from build123d import *

# Parameters (mm, degrees)
F1_DEPTH  = 49
F2_W      = 51.5
F2_H      = 79
F3_DEPTH  = 2
F2_R      = 1.5
F2_R_2    = 4.5
F4_DEPTH  = 7.3
F6_DEPTH  = 2
F8_DEPTH  = 2
F2_R_3    = 5
F9_DEPTH  = 2
F11_DEPTH = 2
F12_W     = 8.5
F12_H     = 55
F13_DEPTH = 40
F14_R     = 1.99999
F15_W     = 2
F15_H     = 19.5
F16_DEPTH = 20
F17_W     = 2
F17_H     = 19.5
F18_DEPTH = 20
F19_R     = 5
F20_DEPTH = 2
F21_R     = 2.5
F22_DEPTH = 7.5
F21_R_2   = 4.5
F23_DEPTH = 2
F25_R     = 2


# Not quite as in the source:
# - a fillet or chamfer that OpenCascade refuses, or shapes differently, is made with other operations: its cross-section is extruded or revolved along the edge and cut away or added
# - a fillet or chamfer is up to 0.001 mm smaller than in the source, because OpenCascade refuses the exact size
# - a feature names something its author has since deleted; it is built from what else it names


with BuildPart() as f1:
    # F0 (on Front) → F1 (new body, symmetric)
    with BuildSketch(Plane.XZ):
        with BuildLine():
            Line((-25, 6.5), (-8.5, 6.5))
            Line((-8.5, 6.5), (-8.5, 0))
            Line((-8.5, 0), (-8.5, -20))
            Line((-8.5, -20), (-6.5, -20))
            Line((-6.5, -20), (-6.5, 0))
            ThreePointArc((-6.5, 0), (2.3181097502, 6.072591472), (4.8465745188, -4.3313641539))
            Line((4.8465745188, -4.3313641539), (6.5, -6))
            Line((6.5, -6), (8.5, -6))
            Line((8.5, -6), (8.5, 0))
            ThreePointArc((8.5, 0), (6.0104076401, 6.0104076401), (0, 8.5))
            Line((0, 8.5), (-25.4288327804, 8.5))
            Line((-25.4288327804, 8.5), (-105.428633061, -27.4597649849))
            Line((-105.428633061, -27.4597649849), (-106.3520655314, -27.8748462039))
            ThreePointArc((-106.3520655314, -27.8748462039), (-110.8598066956, -36.4968976222), (-104.3520655314, -43.7293803221))
            Line((-104.3520655314, -43.7293803221), (-104.3520655314, -42.85))
            Line((-104.3520655314, -42.85), (-104.3520655314, -41.6571435378))
            ThreePointArc((-104.3520655314, -41.6571435378), (-108.9268429391, -35.4298576938), (-104.3520655314, -29.2025718498))
            Line((-104.3520655314, -29.2025718498), (-104.3520655314, -29.1686093911))
            Line((-104.3520655314, -29.1686093911), (-25, 6.5))
        make_face()
    extrude(amount=F1_DEPTH, both=True)

    # F2 (on face) → F3 (cut)
    with BuildSketch(Plane(origin=(-6.6328046362, 0, 14.75602097), x_dir=(0.9120927073, 0, 0.409984016), z_dir=(0.409984016, 0, -0.9120927073))):
        with Locations((-55.3874215775, -0.1)):
            Rectangle(F2_W, F2_H)
    extrude(amount=-F3_DEPTH, mode=Mode.SUBTRACT)

    # F2 (on face) → F4 (join)
    with BuildSketch(Plane(origin=(-6.6328046362, 0, 14.75602097), x_dir=(0.9120927073, 0, 0.409984016), z_dir=(0.409984016, 0, -0.9120927073))):
        with BuildLine():
            Line((-20.1374215775, 40.7130369812), (-20.1374215775, 47.9869630188))
            ThreePointArc((-20.1374215775, 47.9869630188), (-27.2874215775, 44.35), (-20.1374215775, 40.7130369812))
        make_face()
        with Locations((-22.7874215775, 44.35)):
            Circle(F2_R, mode=Mode.SUBTRACT)
        with BuildLine():
            Line((-20.1374215775, -47.5869630188), (-20.1374215775, -40.3130369812))
            ThreePointArc((-20.1374215775, -40.3130369812), (-27.2874215775, -43.95), (-20.1374215775, -47.5869630188))
        make_face()
        with Locations((-22.7874215775, -43.95)):
            Circle(F2_R, mode=Mode.SUBTRACT)
        with Locations((-88.7874215775, -43.95)):
            Circle(F2_R_2)
        with Locations((-88.7874215775, -43.95)):
            Circle(F2_R, mode=Mode.SUBTRACT)
        with Locations((-88.7874215775, 44.35)):
            Circle(F2_R_2)
        with Locations((-88.7874215775, 44.35)):
            Circle(F2_R, mode=Mode.SUBTRACT)
    extrude(amount=F4_DEPTH)

    # F5 (on face) → F6 (join)
    with BuildSketch(Plane.XZ.offset(49)):
        with BuildLine():
            Line((-104.3520655314, -43.7293803221), (-6.5, -20))
            Line((-6.5, -20), (-8.5, -20))
            Line((-8.5, -20), (-8.5, 6.5))
            Line((-8.5, 6.5), (-25, 6.5))
            Line((-25, 6.5), (-104.3520655314, -29.1686093911))
            Line((-104.3520655314, -29.1686093911), (-104.3520655314, -29.2025718498))
            ThreePointArc((-104.3520655314, -29.2025718498), (-108.9268429391, -35.4298576938), (-104.3520655314, -41.6571435378))
            Line((-104.3520655314, -41.6571435378), (-104.3520655314, -43.7293803221))
        make_face()
    extrude(amount=-F6_DEPTH)

    # F7 (on face) → F8 (join)
    with BuildSketch(Plane(origin=(0, 49, 0), x_dir=(-1, 0, 0), z_dir=(0, 1, 0))):
        with BuildLine():
            Line((8.5, -20), (6.5, -20))
            Line((6.5, -20), (104.3520655314, -43.7293803221))
            Line((104.3520655314, -43.7293803221), (104.3520655314, -41.6571435378))
            ThreePointArc((104.3520655314, -41.6571435378), (108.9268429391, -35.4298576938), (104.3520655314, -29.2025718498))
            Line((104.3520655314, -29.2025718498), (104.3520655314, -29.1686093911))
            Line((104.3520655314, -29.1686093911), (25, 6.5))
            Line((25, 6.5), (8.5, 6.5))
            Line((8.5, 6.5), (8.5, -20))
        make_face()
    extrude(amount=-F8_DEPTH)

    # F2 (on face) → F9 (cut)
    with BuildSketch(Plane(origin=(-6.6328046362, 0, 14.75602097), x_dir=(0.9120927073, 0, 0.409984016), z_dir=(0.409984016, 0, -0.9120927073))):
        with Locations((-98.7513456427, 37)):
            Circle(F2_R_3)
    extrude(amount=-F9_DEPTH, mode=Mode.SUBTRACT)

    # F10 (on face) → F11 (cut)
    with BuildSketch(Plane(origin=(0, 49, 0), x_dir=(-1, 0, 0), z_dir=(0, 1, 0))):
        Polygon((63.2235160953, -24.4957862935), (39.5091057066, -13.8362018777), (38.0741616506, -17.0285263531), (61.7885720393, -27.6881107689), align=None)
    extrude(amount=-F11_DEPTH, mode=Mode.SUBTRACT)

    # F12 (on face) → F13 (cut)
    with BuildSketch(Plane.XY.offset(8.5)):
        with Locations((4.25, 0)):
            Rectangle(F12_W, F12_H)
        with Locations((-4.25, 0)):
            Rectangle(F12_W, F12_H)
    extrude(amount=-F13_DEPTH, mode=Mode.SUBTRACT)

    # F14 (radius 2 in the source; OpenCascade refuses exactly that, so slightly less here)
    f14_edges = [f1.edges().sort_by_distance(p)[0] for p in [
        (8.5, 38.25, -6),
        (8.5, -38.25, -6),
    ]]
    fillet(f14_edges, radius=F14_R)

    # F15 (on face) → F16 (join)
    with BuildSketch(Plane(origin=(0, 0, -20), x_dir=(1, 0, 0), z_dir=(0, 0, -1))):
        with Locations((-7.5, 37.25)):
            Rectangle(F15_W, F15_H)
    extrude(amount=F16_DEPTH)

    # F17 (on face) → F18 (join)
    with BuildSketch(Plane(origin=(0, 0, -20), x_dir=(1, 0, 0), z_dir=(0, 0, -1))):
        with Locations((-7.5, -37.25)):
            Rectangle(F17_W, F17_H)
    extrude(amount=F18_DEPTH)

    # F19
    f19_edges = [f1.edges().sort_by_distance(p)[0] for p in [
        (-7.5, 47, -40),
        (-7.5, 27.5, -40),
        (-7.5, -27.5, -40),
        (-7.5, -47, -40),
    ]]
    fillet(f19_edges, radius=F19_R)

    # F2 (on face) → F20 (cut)
    with BuildSketch(Plane(origin=(-6.6328046362, 0, 14.75602097), x_dir=(0.9120927073, 0, 0.409984016), z_dir=(0.409984016, 0, -0.9120927073))):
        with BuildLine():
            ThreePointArc((-100.7513456427, -0.282575695), (-98.7513456427, 9.3), (-96.7513456427, -0.282575695))
            Line((-96.7513456427, -0.282575695), (-96.7513456427, -8.282575695))
            Line((-96.7513456427, -8.282575695), (-95.7513456427, -8.282575695))
            Line((-95.7513456427, -8.282575695), (-95.7513456427, -0.8961524227))
            ThreePointArc((-95.7513456427, -0.8961524227), (-98.7513456427, 10.3), (-101.7513456427, -0.8961524227))
            Line((-101.7513456427, -0.8961524227), (-101.7513456427, -8.282575695))
            Line((-101.7513456427, -8.282575695), (-100.7513456427, -8.282575695))
            Line((-100.7513456427, -8.282575695), (-100.7513456427, -0.282575695))
        make_face()
    extrude(amount=-F20_DEPTH, mode=Mode.SUBTRACT)

    # F21 (on face) → F22 (join)
    with BuildSketch(Plane(origin=(-7.4527726682, 0, 16.5802063845), x_dir=(0.9120927073, 0, 0.409984016), z_dir=(-0.409984016, 0, 0.9120927073))):
        with Locations((-98.7513456427, -4.3)):
            Circle(F21_R)
    extrude(amount=-F22_DEPTH)

    # F21 (on face) → F23 (join)
    with BuildSketch(Plane(origin=(-7.4527726682, 0, 16.5802063845), x_dir=(0.9120927073, 0, 0.409984016), z_dir=(-0.409984016, 0, 0.9120927073))):
        with Locations((-98.7513456427, -4.3)):
            Circle(F21_R_2)
        with Locations((-98.7513456427, -4.3)):
            Circle(F21_R, mode=Mode.SUBTRACT)
        with Locations((-98.7513456427, -4.3)):
            Circle(F21_R)
    extrude(amount=F23_DEPTH)

    # F24: fillet of radius 5 on 1 edges, made by hand

    # F24_s1 → F24_t2 (revolve, cut)
    with BuildSketch(Plane.XZ.offset(4.3)):
        with BuildLine():
            ThreePointArc((-93.4187376781, -22.0613388145), (-95.6311594228, -21.4417982804), (-97.8870765391, -21.877089464))
            Line((-97.8870765391, -21.877089464), (-94.2387057101, -20.2371534))
            Line((-94.2387057101, -20.2371534), (-93.4187376781, -22.0613388145))
        make_face()
    revolve(axis=Axis((-98.3431228928, -4.3, -22.082081472), (-0.409984016, 0, 0.9120927073)), mode=Mode.SUBTRACT)

    # F25
    f25_edges = [f1.edges().sort_by_distance(p)[0] for p in [
        (-96.728507, -4.3, -31.771922),
    ]]
    fillet(f25_edges, radius=F25_R)


solid = f1.part
Read the model definition and answer for the solid it produces. Units are mm, in the model's axes. A direction names the side the tool comes from. Round coordinates to 2 decimals unless told otherwise and drop trailing zeros. Loops run counter-clockwise (first coordinate to the right, second up) from the corner with the lowest first, then second, coordinate; pieces in that order, holes last. Notation, with made-up numbers: (-18.75, 65.25) - (26.25, 65.25) arc R21 ccw to (26.25, 93.25) - close; hole circle Ø11 at (51.5, 71). An arc over 180 degrees is marked (long way). One line per question, with ' | ' between items. Start each with the question number.
Q1. Flat-ended cylindrical pins translate along their axes: pin 1 (5 mm diameter, centred on y = 32.5, z = -10, fed in from +X); pin 2 (1.6 mm diameter, centred on x = -7.5, y = -37, fed in from -Z); pin 3 (1 mm diameter, centred on x = -7, z = -29.5, fed in from +Y); pin 4 (3 mm diameter, centred on y = 30.5, z = -5.5, fed in from +X). Find the tip coordinate at first contact, or state that the pin passes through.
Q2. Find the intervals of material crossed by L1, parallel to X at y = 39, z = 0; L2, parallel to Y at x = -60, z = -16; L3, parallel to Z at x = 0, y = -39, in increasing order.
Q3. For a pull along Z with two mould halves and no side action, classify faces 4 (the cylindrical face through (-26.12, -45.837, 2.051)), 5 (the flat face through (-58, -39.4, -7)), 6 (the cylindrical face through (-94.66, -41.22, -23.73)) as +Z half, -Z half, draft (parallel to the pull), parting line (faces both ways), or undercut.
Q4. For faces 1 (the flat face through (-51.53, 48.01, -19.24)), 2 (the cylindrical face through (-7, 45, -39)), 3 (the flat face through (-27.436, 43.929, 5.405)), determine the directions among +Z, -Z, +X, -X, +Y, -Y from which every point of the face is accessible in a straight line to the end or side of a thin tool.
Q5. Section B-B on x = -42 is taken. Give the vertices of the cut face in (y, z), plus the area to 3 significant figures.
Established:
1) pin 1: x = -6.5 | pin 2: z = -40 | pin 3: y = 47 | pin 4: x = 8.5
2) L1: -8.5 to -6.5, 6.5 to 8.5 | L2: -49 to -47, 47 to 49 | L3: 6.5 to 8.5
3) face 4: undercut | face 5: draft | face 6: parting line
4) face 1: +Y | face 2: -Z, +X, +Y | face 3: none
5) outline: (-49, -28.61) - (-47, -28.61) - (-47, -1.14) - (-39.4, -1.14) - (-39.4, 1.05) - (-49, 1.05) - close; (39.6, -1.14) - (47, -1.14) - (47, -14.96) - (49, -14.96) - (49, 1.05) - (39.6, 1.05) - close; (47, -28.61) - (49, -28.61) - (49, -18.79) - (47, -18.79) - close | area: 144 mm²
